Autodesk Inventor part; units mm, degrees
ref_plane "YZ Plane" through (0, 0, 0) normal (1, 0, 0) x (0, 1, 0)
ref_plane "XZ Plane" through (0, 0, 0) normal (0, 1, 0) x (-1, 0, 0)
ref_plane "XY Plane" through (0, 0, 0) normal (0, 0, 1) x (1, 0, 0)
sketch "Sketch1" plane through (0, 0, 0) normal (0, 1, 0) x (-1, 0, 0)
  arc A0 (9.4829, 2.5433) -> (-8.8962, -4.1533) centre (0, 0) ccw
  line L0 (9.4829, 2.5433) -> (22.3854, -45.5658)
  line L1 (-8.8962, -4.1533) -> (12.1747, -49.2862)
  arc A1 (12.1747, -49.2862) -> (22.3854, -45.5658) centre (17.1171, -46.9788) ccw
  dimension "d0" = 19.636
  dimension "d3" = 5.4545
  dimension "d18" = 50
extrude "Extrusion1" add sketch "Sketch1" along normal blind 1.7
sketch "Sketch2" plane through (0, 1.7, 0) normal (0, 1, 0) x (1, 0, 0)
  arc A0 (-12.1747, 49.2862) -> (-22.3854, 45.5658) centre (-17.1171, 46.9788) ccw
  arc A1 (-9.4829, -2.5433) -> (8.8962, 4.1533) centre (0, 0) ccw
  circle A2 centre (0, 0) radius 1.5
  circle A3 centre (-17.1171, 46.9788) radius 1.5
  circle A4 centre (6.7831, 2.4715) radius 1.5
  circle A5 centre (-6.7831, -2.4715) radius 1.5
  circle A6 centre (-2.4714, 6.7828) radius 1.5
  circle A7 centre (2.4714, -6.7828) radius 1.5
  line L0 (-17.1171, 46.9788) -> (0, 0) construction
  line L1 (-17.1171, 46.9788) -> (-2.4714, 6.7828) construction
  line L2 (0, 0) -> (2.4714, -6.7828) construction
  line L3 (-6.7831, -2.4715) -> (0, 0) construction
  line L4 (0, 0) -> (6.7831, 2.4715) construction
  dimension "d4" = 3
  dimension "d5" = 3
  dimension "d6" = 3
  dimension "d7" = 3
  dimension "d12" = 3
  dimension "d13" = 3
  dimension "d19" = 7.219
  dimension "d20" = 7.2193
  dimension "d21" = 7.2193
  dimension "d22" = 7.219
extrude "Extrusion2" cut sketch "Sketch2" against normal blind 1.7
sketch "Sketch3" plane through (0, 1.7, 0) normal (0, 1, 0) x (1, 0, 0)
  circle A0 centre (0, 0) radius 1.5
  circle A1 centre (0, 0) radius 3
  dimension "d25" = 6
extrude "Extrusion3" cut sketch "Sketch3" against normal through all contours A0 | A1
equation "\"BendRadius\" = Thickness"
equation "\"BendReliefWidth\" = Thickness"
equation "\"BendReliefDepth\" = 0.5 * Thickness"
equation "\"CornerReliefSize\" = 4 * Thickness"
equation "\"MinimumRemnant\" = 2 * Thickness"
equation "\"TransitionRadius\" = BendRadius"
equation "\"JacobiRadiusSize\" = BendRadius"
equation "\"GapSize\" = Thickness"
properties part number "A1P1"
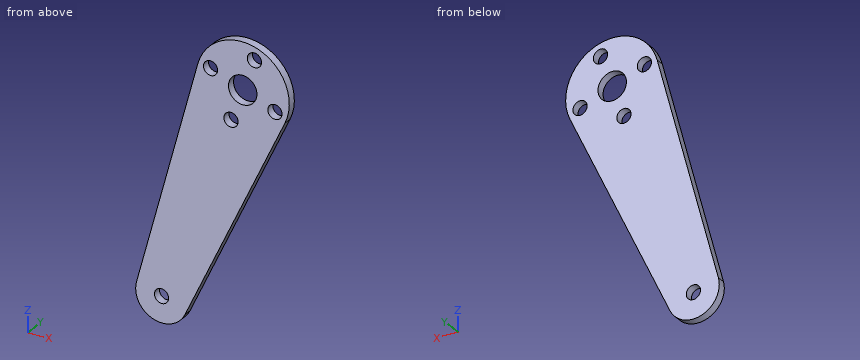
Check sheet for the modelled part. Datum: model origin and axes. Units: mm. Give positions to 0.01 mm unless a question says otherwise; leave off trailing zeros. Order: outer loops, then holes, each group sorted by start corner. A loop starts at its lowest first (then second) coordinate and runs counter-clockwise, first axis right, second up. Notation, with made-up numbers: M -35.5,-3 L -18.5,-3 A30 cw -18.5,31 Z; hole C 55.5,67 d5. An arc over 180 degrees is marked long. Answer in a Markdown table with one row per item. Add a question column.
Q1. Sectioned sample at A-A, the plane z = 0. Record the boundary of the cut face in (x, y) (3 decimals).
Q2. Sectioned sample at B-B, the plane x = 0. Record the boundary of the cut face in (y, z).
Q3. Gauge pin test, flat end, axial feed: pin 1 Ø2.5 at (x, z) = (2.47, 6.78) entering from +Y. Record the tip position at first contact, or that the pin passes through.
Q4. Sectioned sample at D-D, the plane z = -11. Record the boundary of the cut face in (x, y).
Q5. Sectioned sample at C-C, the plane y = 0.65. Record the boundary of the cut face in (x, z).
Q6. Thickness scan on L1, parallel to X at y = 0.3, z = -1.5; L2, parallel to Z at x = 2.5, y = 1.05; L3, parallel to Z at x = 8, y = 0.9. Record the ranges inside material, lowest first.
Verdict:
| question | item | result |
|---|---|---|
| 1 | outline | M -10.165,0 L -3,0 L -3,1.7 L -10.165,1.7 Z; M 3,0 L 9.818,0 L 9.818,1.7 L 3,1.7 Z |
| 2 | outline | M 0,-23.21 L 1.7,-23.21 L 1.7,-3 L 0,-3 Z; M 0,3 L 1.7,3 L 1.7,9.82 L 0,9.82 Z |
| 3 | pin 1 | through |
| 4 | outline | M -13.12,0 L 5.7,0 L 5.7,1.7 L -13.12,1.7 Z |
| 5 | outline | M -22.39,-45.57 A5.45 ccw -12.17,-49.29 L 8.9,-4.15 A9.82 ccw long -9.48,2.54 Z; hole C -17.12,-46.98 d3; hole C -6.78,2.47 d3; hole C -2.47,-6.78 d3; hole C 0,0 d6; hole C 2.47,6.78 d3; hole C 6.78,-2.47 d3 |
| 6 | L1 | -10.57 to -2.6, 2.6 to 5.64, 7.93 to 9.7 |
| 6 | L2 | -17.85 to -1.66, 1.66 to 5.28, 8.28 to 9.49 |
| 6 | L3 | -6.07 to -3.35, -1.59 to 5.69 |
